from build123d import *

# Parameters (mm, degrees)
SKETCH2_R           = 50
BOSS_EXTRUDE1_DEPTH = 30
SHELL1_T            = -3
CUT_EXTRUDE3_DEPTH  = 27


with BuildPart() as part:
    # Sketch2 → Boss-Extrude1 (new body)
    with BuildSketch(Plane(origin=(0, 0, 0), x_dir=(1, 0, 0), z_dir=(0, 1, 0))):
        Polygon((-35.583006561, -114.820946016), (114.820946016, -35.583006561), (35.583006561, 114.820946016), (-114.820946016, 35.583006561), align=None)
        with Locations(Location((0, 0, 0), (0, 0, 270))):
            Circle(SKETCH2_R, mode=Mode.SUBTRACT)
    extrude(amount=BOSS_EXTRUDE1_DEPTH)

    # Shell1
    shell1_openings = [part.faces().sort_by_distance(p)[0] for p in [
        (38.105232938, 30, 72.328706262),
    ]]
    offset(amount=SHELL1_T, openings=shell1_openings, kind=Kind.INTERSECTION)

    # Sketch7 → Cut-Extrude3 (cut)
    with BuildSketch(Plane(origin=(0, 30, 0), x_dir=(1, 0, 0), z_dir=(0, 1, 0))):
        Polygon((79.539371783, 24.949716157), (82.193559182, 26.348032736), (68.210393395, 52.88990672), (65.556205997, 51.491590141), align=None)
        Polygon((51.491590141, -65.556205997), (24.949716157, -79.539371783), (26.348032736, -82.193559182), (52.88990672, -68.210393395), align=None)
        Polygon((-65.556205997, -51.491590141), (-79.539371783, -24.949716157), (-82.193559182, -26.348032736), (-68.210393395, -52.88990672), align=None)
        Polygon((-51.491590141, 65.556205997), (-24.949716157, 79.539371783), (-26.348032736, 82.193559182), (-52.88990672, 68.210393395), align=None)
    extrude(amount=-CUT_EXTRUDE3_DEPTH, mode=Mode.SUBTRACT)


solid = part.part
For this review, take the finished solid that the model builds, in its own axes (mm). A direction names the side the tool comes from. Coordinates: 2 decimals unless noted, no trailing zeros. Order: outer loops, then holes, each group sorted by start corner. A loop starts at its lowest first (then second) coordinate and runs counter-clockwise, first axis right, second up. Notation, with made-up numbers: (-30.75, -14) - (-21.75, -14) arc R20 cw to (-21.75, 9) - close; hole circle Ø6 at (29, 21). An arc over 180 degrees is marked (long way). Use one line per item in the form item = value.
Q1. Consider section B-B (x = 14.5). Give the boundary of the cut face in (y, z).
Checked values:
outline = (0, -103.71) - (30, -103.71) - (30, -100.32) - (3, -100.32) - (3, -50.98) - (30, -50.98) - (30, -47.85) - (0, -47.85) - close; (0, 47.85) - (30, 47.85) - (30, 50.98) - (3, 50.98) - (3, 85.04) - (30, 85.04) - (30, 88.44) - (0, 88.44) - close
Q2. Draft analysis for pull direction Z (two halves, no side actions). For faces 1 (the flat face through (75.757, 1.457, -38.566)), 2 (the cylindrical face through (15.02, 14.79, 47.69)), 3 (the flat face through (97, 30, 42)), 4 (the flat face through (38.566, 1.457, 75.757)), state which applies: +Z half, -Z half, draft (parallel to the pull), parting line (faces both ways), or undercut.
Checked values:
face_1 = -Z half
face_2 = undercut
face_3 = draft
face_4 = +Z half
Q3. Consider section C-C (z = 19.5). Give the boundary of the cut face in (x, y).
Checked values:
outline = (-85.8, 0) - (-46.04, 0) - (-46.04, 30) - (-49.28, 30) - (-49.28, 3) - (-82.41, 3) - (-82.41, 30) - (-85.8, 30) - close; (46.04, 0) - (106.35, 0) - (106.35, 30) - (102.96, 30) - (102.96, 3) - (49.28, 3) - (49.28, 30) - (46.04, 30) - close
Q4. For P1, Ø1, axis at y = 12, z = 83.5, coming from the +X side; P2, Ø5, axis at y = 20, z = -41, coming from the -X side; P3, Ø3, axis at x = 54.5, y = 26, coming from the -Z side; P4, Ø2, axis at x = 32.5, z = -79, coming from the -Y side, all flat-tipped, find the tip position at first contact; note any pin that passes through.
Checked values:
P1 = 24.82
P2 = -109.28
P3 = -81.76
P4 = 0
Q5. For probe 1 along X at (y, z) = (26.25, -33.5); probe 2 along X at (y, z) = (23.5, 18.5); probe 3 along X at (y, z) = (11.5, -11) (3 decimals), list the stretches that pass through material, from the lowest coordinate up. Write a range as from..to.
Checked values:
probe_1 = -113.72..-110.33, -41.07..-37.12, 37.12..41.07
probe_2 = -86.33..-82.94, -49.67..-46.45, 46.45..49.67, 102.43..105.82
probe_3 = -101.87..-98.479, -51.846..-48.775, 48.775..51.846, 86.889..90.279
Q6. Consider section D-D (z = -71). Give the boundary of the cut face in (x, y), then the cut area to 3 significant figures.
Checked values:
outline = (-47.59, 0) - (58.67, 0) - (58.67, 30) - (55.28, 30) - (55.28, 3) - (-47.59, 3) - close
area = 410 mm2
Q7. For faces 5 (the flat face through (-5.1, 16.31, 95.37)), 6 (the flat face through (-75.757, 1.457, 38.566)), list the 3-axis set-ups (+Z, -Z, +X, -X, +Y, -Y) from which the entire face can be reached by the end or side of a thin tool; tool diameter is ignored.
Checked values:
face_5 = +Y
face_6 = +Z, -X, +Y, -Y
Q8. Consider section A-A (y = 12). Give the boundary of the cut face in (x, z).
Checked values:
outline = (-114.82, -35.58) - (-52.89, -68.21) - (-51.49, -65.56) - (-110.77, -34.33) - (-79.54, 24.95) - (-82.19, 26.35) - close; (-68.21, 52.89) - (-65.56, 51.49) - (-34.33, 110.77) - (24.95, 79.54) - (26.35, 82.19) - (-35.58, 114.82) - close; circle Ø106 at (0, 0); (-26.35, -82.19) - (35.58, -114.82) - (68.21, -52.89) - (65.56, -51.49) - (34.33, -110.77) - (-24.95, -79.54) - close; (51.49, 65.56) - (110.77, 34.33) - (79.54, -24.95) - (82.19, -26.35) - (114.82, 35.58) - (52.89, 68.21) - close; hole circle Ø100 at (0, 0)
